Input: part model. Units: mm. Frame: model coordinates. A direction names the side the tool comes from. Round coordinates to 2 decimals unless told otherwise and drop trailing zeros. Write each loop counter-clockwise with the first axis right and the second up, starting at its lowest first coordinate (ties: lowest second). Pieces come first, ordered by that corner, then holes. Notation, with made-up numbers: M 48,23.25 L 104,23.25 A22 cw 104,44.25 Z; hole C 39.5,-5 d7. An arc over 180 degrees is marked long. Answer as CSV lines item,"result". Start each with the question number.
```python
from build123d import *

# Parameters (mm, degrees)
F0_R      = 4.325
F1_DEPTH  = 15
F4_R      = 4.5
F4_R_2    = 3
F5_DEPTH  = 2
F6_R      = 4.5
F6_R_2    = 3
F7_DEPTH  = 2
F8_SIZE   = 0.5
F9_R      = 0.5
F10_R     = 2
F11_DEPTH = 5


with BuildPart() as f1:
    # F0 (on Front) → F1 (new body)
    with BuildSketch(Plane.XZ):
        Circle(F0_R)
    extrude(amount=-F1_DEPTH)

    # F4 (on offset) → F5 (cut)
    with BuildSketch(Plane.XZ.offset(-3)):
        Circle(F4_R)
        Circle(F4_R_2, mode=Mode.SUBTRACT)
    extrude(amount=-F5_DEPTH, mode=Mode.SUBTRACT)

    # F6 (on offset) → F7 (cut)
    with BuildSketch(Plane.XZ.offset(-10)):
        Circle(F6_R)
        Circle(F6_R_2, mode=Mode.SUBTRACT)
    extrude(amount=-F7_DEPTH, mode=Mode.SUBTRACT)

    # F8
    f8_edges = [f1.edges().sort_by_distance(p)[0] for p in [
        (-4.325, 0, 0),
        (-4.325, 15, 0),
    ]]
    chamfer(f8_edges, length=F8_SIZE)

    # F9
    f9_edges = [f1.edges().sort_by_distance(p)[0] for p in [
        (-3, 5, 0),
        (-3, 12, 0),
        (-3, 10, 0),
        (-3, 3, 0),
    ]]
    fillet(f9_edges, radius=F9_R)

    # F10 (on face) → F11 (cut)
    with BuildSketch(Plane(origin=(0, 15, 0), x_dir=(-1, 0, 0), z_dir=(0, 1, 0))):
        Circle(F10_R)
    extrude(amount=-F11_DEPTH, mode=Mode.SUBTRACT)


solid = f1.part
```
Item 1: Cut plane B-B, the plane x = 3.25. Give the number of separate pieces and of enclosed holes in the cut face, plus the area to 3 significant figures.
Item 2: Cut plane A-A, the plane y = 8.75. Return loops of the section in (x, z) (3 decimals).
Item 3: Cut plane C-C, the plane y = 11.75. Return loops of the section in (x, z).
Item 4: Draft query along X for faces 1 (the face through (-3, 11, 0)), 2 (the face through (4, 5, 0)), 3 (the face through (0, 10, 0)). Return one class per face: +X half, -X half, draft (parallel to the pull), parting line (faces both ways), or undercut.
Item 5: Line query: line 1 (Y direction, x = -2.25, z = 2.75); line 2 (Z direction, x = 0, y = 12.85) (3 decimals); line 3 (Y direction, x = 3, z = 2.75). Output: solid intervals per line, ascending. Write a range as [from, to].
Item 6: Access query for faces 4 (the face through (0, 13, -2)), 5 (the face through (4.125, 13.232, 1.299)), 6 (the face through (4, 10, 0)). Directions: +Z, -Z, +X, -X, +Y, -Y. A direction counts if a zero-diameter tool reaches every point of the face in a straight line with its end or side. Return the directions, or none.
Item 7: Pin query (flat end, axial travel): pin 1 Ø2 at (x, z) = (-1, -1) entering from +Y; pin 2 Ø4 at (y, z) = (6.5, 3.5) entering from +X; pin 3 Ø5 at (y, z) = (10.5, 3) entering from +X; pin 4 Ø2 at (x, y) = (3, 11.5) entering from -Z. Return the tip coordinate at first contact, or that it passes through.
Results list:
1,separate pieces,"3"
1,enclosed holes,"0"
1,area,"62.3 mm²"
2,outline,"C 0,0 d8.65"
3,outline,"C 0,0 d6.13; hole C 0,0 d4"
4,face 1,"parting line"
4,face 2,"draft"
4,face 3,"undercut"
5,line 1,"[0, 3], [5, 10], [12, 15]"
5,line 2,"[-4.325, -2], [2, 4.325]"
5,line 3,"[0.24, 3], [5, 10], [12, 14.76]"
6,face 4,"+Y"
6,face 5,"+Y, -Y"
6,face 6,"none"
7,pin 1,"y = 15"
7,pin 2,"x = 4.06"
7,pin 3,"x = 4.29"
7,pin 4,"z = -3.76"
